from build123d import *

# Parameters (mm, degrees)
SKETCH1_W           = 10
SKETCH1_H           = 10
SKETCH1_W_2         = 8
SKETCH1_H_2         = 8
BOSS_EXTRUDE1_DEPTH = 140
SKETCH2_R           = 2.025
CUT_EXTRUDE1_DEPTH  = 141.445719052
SKETCH3_R           = 2.025
CUT_EXTRUDE2_DEPTH  = 141.445719052
SKETCH4_R           = 2.025
CUT_EXTRUDE3_DEPTH  = 141.445719052


with BuildPart() as part:
    # Sketch1 → Boss-Extrude1 (new body)
    with BuildSketch(Plane.XY):
        Rectangle(SKETCH1_W, SKETCH1_H)
        Rectangle(SKETCH1_W_2, SKETCH1_H_2, mode=Mode.SUBTRACT)
    extrude(amount=BOSS_EXTRUDE1_DEPTH)

    # Sketch2 → Cut-Extrude1 (cut, through all)
    with BuildSketch(Plane(origin=(5, 0, 0), x_dir=(0, 0, -1), z_dir=(1, 0, 0))):
        with Locations(Location((-5, 0, 0), (0, 0, 90))):
            Circle(SKETCH2_R)
    extrude(amount=-CUT_EXTRUDE1_DEPTH, mode=Mode.SUBTRACT)

    # Sketch3 → Cut-Extrude2 (cut, through all)
    with BuildSketch(Plane(origin=(5, 0, 0), x_dir=(0, 0, -1), z_dir=(1, 0, 0))):
        with Locations(Location((-75, 0, 0), (0, 0, 90))):
            Circle(SKETCH3_R)
        with Locations(Location((-55, 0, 0), (0, 0, 90))):
            Circle(SKETCH3_R)
    extrude(amount=-CUT_EXTRUDE2_DEPTH, mode=Mode.SUBTRACT)

    # Sketch4 → Cut-Extrude3 (cut, through all)
    with BuildSketch(Plane(origin=(5, 0, 0), x_dir=(0, 0, -1), z_dir=(1, 0, 0))):
        with Locations(Location((-135, 0, 0), (0, 0, 90))):
            Circle(SKETCH4_R)
        with Locations(Location((-95, 0, 0), (0, 0, 90))):
            Circle(SKETCH4_R)
    extrude(amount=-CUT_EXTRUDE3_DEPTH, mode=Mode.SUBTRACT)


solid = part.part
Source: CAD feature listing. Evaluate the final solid. Frame: model axes, mm. A direction names the side the tool comes from. Round coordinates to 2 decimals unless told otherwise and drop trailing zeros. Order: outer loops, then holes, each group sorted by start corner. A loop starts at its lowest first (then second) coordinate and runs counter-clockwise, first axis right, second up. Notation, with made-up numbers: (70, 89.5) - (74, 89.5) arc R15 ccw to (74, 104.5) - close; hole circle Ø10 at (23, 28.25). An arc over 180 degrees is marked (long way). Use a Markdown table: item, result. Add a question column.
1. Section query B-B (z = 95). Return the cut outline in (x, y) (3 decimals).
2. Section query D-D (y = 0). Give the number of separate pieces and of enclosed holes in the cut face, then the cut area to 4 significant figures.
3. First-contact query: pin 1 (5.5 mm diameter, centred on y = 0, z = 55, fed in from +X). Flat tip, straight axial feed; report the tip coordinate or a pass-through.
4. Section query C-C (z = 50.5). Return the cut outline in (x, y).
5. Line query: probe 1 along Z at (x, y) = (4.5, 0) (3 decimals); probe 2 along X at (y, z) = (-1, 33). Output: solid intervals per line, ascending.
6. Section query A-A (x = -1). Return the cut outline in (y, z), then the cut area to 3 significant figures.
7. Mould query, pull axis X, two halves, no side actions, for faces 1 (the flat face through (5, 0, 69)), 2 (the flat face through (-5, 0, 69)), 3 (the flat face through (0, -5, 69)), 4 (the flat face through (0, 4, 69)). Classes: +X half, -X half, draft (parallel to the pull), parting line (faces both ways), or undercut.
8. Set-up query: faces 5 (the cylindrical face through (-4.49, -0.26, 97.01)), 6 (the flat face through (-4, 0, 69)). Return all of +Z, -Z, +X, -X, +Y, -Y with unobstructed straight access to the full face (end or side cutting, diameter ignored); none if empty.
Derived:
| question | item | result |
|---|---|---|
| 1 | outline | (-5, -5) - (5, -5) - (5, -2.025) - (4, -2.025) - (4, -4) - (-4, -4) - (-4, -2.025) - (-5, -2.025) - close; (-5, 2.025) - (-4, 2.025) - (-4, 4) - (4, 4) - (4, 2.025) - (5, 2.025) - (5, 5) - (-5, 5) - close |
| 2 | separate pieces | 12 |
| 2 | enclosed holes | 0 |
| 2 | area | 239.5 mm2 |
| 3 | pin 1 | x = 5 |
| 4 | outline | (-5, -5) - (5, -5) - (5, 5) - (-5, 5) - close; hole (-4, -4) - (4, -4) - (4, 4) - (-4, 4) - close |
| 5 | probe 1 | 0 to 2.975, 7.025 to 52.975, 57.025 to 72.975, 77.025 to 92.975, 97.025 to 132.975, 137.025 to 140 |
| 5 | probe 2 | -5 to -4, 4 to 5 |
| 6 | outline | (-5, 0) - (-4, 0) - (-4, 140) - (-5, 140) - close; (4, 0) - (5, 0) - (5, 140) - (4, 140) - close |
| 6 | area | 280 mm2 |
| 7 | face 1 | +X half |
| 7 | face 2 | -X half |
| 7 | face 3 | draft |
| 7 | face 4 | undercut |
| 8 | face 5 | +X, -X |
| 8 | face 6 | +Z, -Z |
